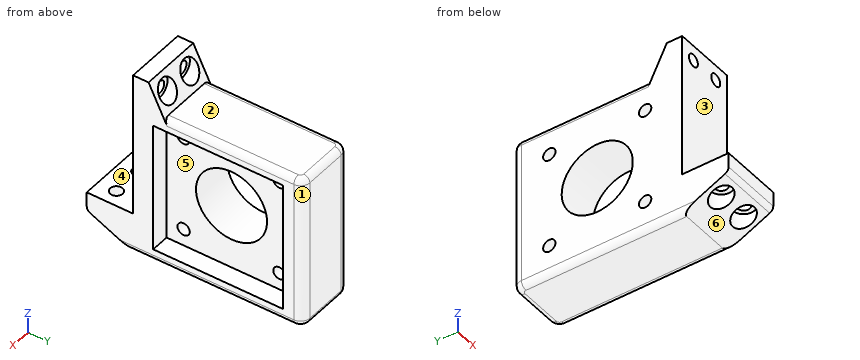
```python
from build123d import *

# Parameters (mm, degrees)
SKETCH1_W           = 20
SKETCH1_H           = 50
BOSS_EXTRUDE1_DEPTH = 70
SKETCH2_R           = 2
SKETCH2_R_2         = 11.5
CUT_EXTRUDE2_DEPTH  = 60
SKETCH4_W           = 37
SKETCH4_H           = 15
CUT_EXTRUDE3_DEPTH  = 60
SKETCH8_R           = 2
CUT_EXTRUDE5_DEPTH  = 15
SKETCH9_W           = 42
SKETCH9_H           = 42
CUT_EXTRUDE6_DEPTH  = 6
CUT_EXTRUDE8_DEPTH  = 30
SKETCH12_W          = 20
SKETCH12_H          = 5
BOSS_EXTRUDE2_DEPTH = 10
BOSS_EXTRUDE3_DEPTH = 20
SKETCH15_R          = 2
CUT_EXTRUDE9_DEPTH  = 10
SKETCH17_R          = 3.5
CUT_EXTRUDE11_DEPTH = 8
SKETCH18_R          = 3.5
CUT_EXTRUDE12_DEPTH = 50
FILLET2_R           = 3
FILLET3_R           = 3
FILLET4_R           = 2
FILLET5_R           = 2
FILLET6_R           = 2


with BuildPart() as part:
    # Sketch1 → Boss-Extrude1 (new body)
    with BuildSketch(Plane(origin=(0, 0, 0), x_dir=(1, 0, 0), z_dir=(0, 1, 0))):
        with Locations((-10, -25)):
            Rectangle(SKETCH1_W, SKETCH1_H)
    extrude(amount=BOSS_EXTRUDE1_DEPTH)

    # Sketch2 → Cut-Extrude2 (cut)
    with BuildSketch(Plane(origin=(0, 0, 0), x_dir=(0, 0, -1), z_dir=(1, 0, 0))):
        with Locations((-9.5, 58)):
            Circle(SKETCH2_R)
        with Locations((-25, 42.5)):
            Circle(SKETCH2_R_2)
        with Locations((-9.5, 27)):
            Circle(SKETCH2_R)
        with Locations((-40.5, 27)):
            Circle(SKETCH2_R)
        with Locations((-40.5, 58)):
            Circle(SKETCH2_R)
    extrude(amount=-CUT_EXTRUDE2_DEPTH, mode=Mode.SUBTRACT)

    # Sketch4 → Cut-Extrude3 (cut)
    with BuildSketch(Plane(origin=(0, 0, 0), x_dir=(0, 0, -1), z_dir=(1, 0, 0))):
        with Locations((-31.5, 7.5)):
            Rectangle(SKETCH4_W, SKETCH4_H)
    extrude(amount=-CUT_EXTRUDE3_DEPTH, mode=Mode.SUBTRACT)

    # Sketch8 → Cut-Extrude5 (cut)
    with BuildSketch(Plane(origin=(0, 0, 0), x_dir=(-1, 0, 0), z_dir=(0, 0, -1))):
        with Locations((15, 6)):
            Circle(SKETCH8_R)
        with Locations((5, 6)):
            Circle(SKETCH8_R)
    extrude(amount=-CUT_EXTRUDE5_DEPTH, mode=Mode.SUBTRACT)

    # Sketch9 → Cut-Extrude6 (cut)
    with BuildSketch(Plane(origin=(0, 0, 0), x_dir=(0, 0, -1), z_dir=(1, 0, 0))):
        with Locations((-25, 42.5)):
            Rectangle(SKETCH9_W, SKETCH9_H)
    extrude(amount=-CUT_EXTRUDE6_DEPTH, mode=Mode.SUBTRACT)

    # Sketch11 → Cut-Extrude8 (cut)
    with BuildSketch(Plane(origin=(0, 0, 0), x_dir=(0, 0, -1), z_dir=(1, 0, 0))):
        Polygon((-7, 0), (0, 0), (0, 15), align=None)
    extrude(amount=-CUT_EXTRUDE8_DEPTH, mode=Mode.SUBTRACT)

    # Sketch12 → Boss-Extrude2 (add)
    with BuildSketch(Plane.XY.offset(50)):
        with Locations((-10, 17.5)):
            Rectangle(SKETCH12_W, SKETCH12_H)
    extrude(amount=BOSS_EXTRUDE2_DEPTH)

    # Sketch14 → Boss-Extrude3 (add)
    with BuildSketch(Plane(origin=(0, 0, 0), x_dir=(0, 0, -1), z_dir=(1, 0, 0))):
        Polygon((-50, 20), (-60, 20), (-50, 25), align=None)
    extrude(amount=-BOSS_EXTRUDE3_DEPTH)

    # Sketch15 → Cut-Extrude9 (cut)
    with BuildSketch(Plane(origin=(0, 15, 0), x_dir=(-1, 0, 0), z_dir=(0, -1, 0))):
        with Locations(Location((5, -55, 0), (0, 0, 90))):
            Circle(SKETCH15_R)
        with Locations(Location((15, -55, 0), (0, 0, 90))):
            Circle(SKETCH15_R)
    extrude(amount=-CUT_EXTRUDE9_DEPTH, mode=Mode.SUBTRACT)

    # Sketch17 → Cut-Extrude11 (cut)
    with BuildSketch(Plane(origin=(0, 0, 0), x_dir=(-1, 0, 0), z_dir=(0, 0, -1))):
        with Locations((15, 6)):
            Circle(SKETCH17_R)
        with Locations((5, 6)):
            Circle(SKETCH17_R)
    extrude(amount=-CUT_EXTRUDE11_DEPTH, mode=Mode.SUBTRACT)

    # Sketch18 → Cut-Extrude12 (cut)
    with BuildSketch(Plane(origin=(0, 70, 0), x_dir=(1, 0, 0), z_dir=(0, 1, 0))):
        with Locations(Location((-15, -55, 0), (0, 0, 270))):
            Circle(SKETCH18_R)
        with Locations(Location((-5, -55, 0), (0, 0, 270))):
            Circle(SKETCH18_R)
    extrude(amount=-CUT_EXTRUDE12_DEPTH, mode=Mode.SUBTRACT)

    # Fillet2
    fillet2_edges = [part.edges().sort_by_distance(p)[0] for p in [
        (0, 70, 25),
    ]]
    fillet(fillet2_edges, radius=FILLET2_R)

    # Fillet3
    fillet3_edges = [part.edges().sort_by_distance(p)[0] for p in [
        (-20, 70, 25),
    ]]
    fillet(fillet3_edges, radius=FILLET3_R)

    # Fillet4
    fillet4_edges = [part.edges().sort_by_distance(p)[0] for p in [
        (0, 46, 50),
        (-0.878679656, 69.121320344, 50),
        (-10, 70, 50),
        (-20, 46, 50),
        (-19.121320344, 69.121320344, 50),
    ]]
    fillet(fillet4_edges, radius=FILLET4_R)

    # Fillet5
    fillet5_edges = [part.edges().sort_by_distance(p)[0] for p in [
        (-10, 70, 0),
        (0, 41, 0),
        (-0.878679656, 69.121320344, 0),
        (-20, 41, 0),
        (-19.121320344, 69.121320344, 0),
    ]]
    fillet(fillet5_edges, radius=FILLET5_R)

    # Fillet6
    fillet6_edges = [part.edges().sort_by_distance(p)[0] for p in [
        (-10, 0, 7),
    ]]
    fillet(fillet6_edges, radius=FILLET6_R)


solid = part.part
```
The listing builds one solid part. Answer for the finished solid, in the listing's coordinates (mm). Face numbers are marked on the shaded views. A direction names the side the tool comes from. Round coordinates to 2 decimals unless told otherwise and drop trailing zeros. Loops run counter-clockwise (first coordinate to the right, second up) from the corner with the lowest first, then second, coordinate; pieces in that order, holes last. Notation, with made-up numbers: (67, -9.75) - (115, -9.75) arc R16 ccw to (115, -5.75) - close; hole circle Ø4 at (39.5, 83). An arc over 180 degrees is marked (long way). Use one line per item in the form item = value. Start each with the question number.
1. The part is cut by section C-C on y = 42.5. Determine the outline of the cut face in (x, z), then the cut area to 3 significant figures.
2. The part is cut by section D-D on x = -9.5. Determine the outline of the cut face in (y, z).
3. For a pull along Y with two mould halves and no side action, classify the marked faces 4, 5 and 6 as pulls with the +Y half, pulls with the -Y half, needs draft (parallel to the pull), parting line crosses it, or undercut.
4. The part is cut by section A-A on z = 9.5. Determine the outline of the cut face in (x, y), then the cut area to 3 significant figures.
5. Given pin 1 Ø6.5 at (x, y) = (-15, 6) entering from -Z; pin 2 Ø1.8 at (x, z) = (-1.5, 26.5) entering from -Y; pin 3 Ø5 at (y, z) = (58, 9.5) entering from +X; pin 4 Ø3 at (y, z) = (22.5, 35) entering from +X, each flat-ended and moving along its own axis, determine where each tip first touches the part or whether it passes through.
6. A tool of negligible diameter and unlimited length cuts with its end or side. For the marked faces 1, 2 and 3, from which of +Z, -Z, +X, -X, +Y, -Y can it reach the whole face along a straight path? Write none if from no direction.
7. The part is cut by section B-B on x = -5. Give the number of separate pieces and of enclosed holes in the cut face, then the cut area to 3 significant figures.
8. Consider line 1 (X direction, y = 57, z = 43); line 2 (Z direction, x = -5.5, y = 38.5); line 3 (Y direction, x = -10, z = 45). Determine where each line is inside the solid, lowest interval first. Write a range as [from, to].
Geometry check:
q1.outline = (-20, 2) arc R2 ccw to (-18, 0) - (-2, 0) arc R2 ccw to (0, 2) - (0, 4) - (-6, 4) - (-6, 13.5) - (-20, 13.5) - close; (-20, 36.5) - (-6, 36.5) - (-6, 46) - (0, 46) - (0, 48) arc R2 ccw to (-2, 50) - (-18, 50) arc R2 ccw to (-20, 48) - close
q1.area = 423 mm^2
q2.outline = (0, 8.27) arc R2 ccw to (1.15, 6.46) - (15, 0) - (68, 0) arc R2 ccw to (70, 2) - (70, 48) arc R2 ccw to (68, 50) - (25, 50) - (20, 60) - (15, 60) - (15, 13) - (0, 13) - close; hole circle Ø4 at (27, 9.5); hole circle Ø4 at (27, 40.5); hole circle Ø23 at (42.5, 25); hole circle Ø4 at (58, 9.5); hole circle Ø4 at (58, 40.5)
q3.face_4 = needs draft
q3.face_5 = undercut
q3.face_6 = pulls with the -Y half
q4.outline = (-20, 0) - (0, 0) - (0, 21.5) - (-6, 21.5) - (-6, 25) - (-20, 25) - close; (-20, 29) - (-6, 29) - (-6, 56) - (-20, 56) - close; (-20, 60) - (-6, 60) - (-6, 63.5) - (0, 63.5) - (0, 67) arc R3 ccw to (-3, 70) - (-17, 70) arc R3 ccw to (-20, 67) - close; hole circle Ø4 at (-15, 6); hole circle Ø4 at (-5, 6)
q4.area = 1,010 mm^2
q5.pin_1 = 8
q5.pin_2 = 15
q5.pin_3 = -6
q5.pin_4 = 0
q6.face_1 = +Z, -Z, +X, +Y
q6.face_2 = +Z, +X, -X, +Y
q6.face_3 = +Z, +X, -X, -Y
q7.separate_pieces = 3
q7.enclosed_holes = 1
q7.area = 1,120 mm^2
q8.line_1 = [-20, -6]
q8.line_2 = [0, 4], [46, 50]
q8.line_3 = [15, 70]
